Source: CAD feature listing. Evaluate the final solid. Frame: model axes, mm. A direction names the side the tool comes from. Round coordinates to 2 decimals unless told otherwise and drop trailing zeros. Loops run counter-clockwise (first coordinate to the right, second up) from the corner with the lowest first, then second, coordinate; pieces in that order, holes last. Notation, with made-up numbers: (50.5, -39) -> (57.5, -39) arc R28 cw to (57.5, -8) -> close; hole circle Ø8 at (16.5, 84). An arc over 180 degrees is marked (long way). Put each result on its own line as item: value. Start each with the question number.
1. Cut plane B-B (z = -37.5). Return the cut outline in (x, y).
2. Cut plane A-A (x = -4.25). Return the cut outline in (y, z), then the cut area to 3 significant figures.
3. Contact query for flat-ended pins moving along their axis: pin 1 (5 mm diameter, centred on x = -16.5, y = 26, fed in from -Z); pin 2 (9 mm diameter, centred on x = -9, z = -22, fed in from +Y); pin 3 (10 mm diameter, centred on x = -9, y = 17.5, fed in from +Z); pin 4 (4 mm diameter, centred on x = -13, z = -43, fed in from +Y). Output: stop coordinate, or through.
4. Cut plane C-C (z = -43). Return the cut outline in (x, y), then the cut area to 3 significant figures.
5. Set-up query: faces 1 (the flat face through (-10, 18, -40)), 2 (the cylindrical face through (-9.67, 43.21, -32.38)), 3 (the flat face through (-10, 18, 0)). Return all of +Z, -Z, +X, -X, +Y, -Y with unobstructed straight access to the full face (end or side cutting, diameter ignored); none if empty.
6. Material intervals for L1, parallel to X at y = 29.5, z = 4.75; L2, parallel to Y at x = -1, z = -36; L3, parallel to Y at x = -1.25, z = 1, sorted ascending.
7. Cut plane D-D (x = -10). Return the cut outline in (y, z), then the cut area to 3 significant figures.
Autodesk Inventor part; units mm, degrees
ref_plane "YZ Plane" through (0, 0, 0) normal (1, 0, 0) x (0, 1, 0)
ref_plane "XZ Plane" through (0, 0, 0) normal (0, 1, 0) x (-1, 0, 0)
ref_plane "XY Plane" through (0, 0, 0) normal (0, 0, 1) x (1, 0, 0)
sketch "Sketch1" plane through (0, 0, 0) normal (1, 0, 0) x (0, 1, 0)
  line L0 (0, 0) -> (40.5, 0)
  line L1 (40.5, 0) -> (40.5, -40)
  line L2 (40.5, -40) -> (0, -40)
  line L3 (0, -40) -> (0, 0)
  line L4 (46, -27.4) -> (40.5, -27.4)
  line L5 (40.5, -27.4) -> (40.5, -32.4)
  line L6 (40.5, -32.4) -> (46, -32.4)
  line L7 (46, -32.4) -> (46, -27.4)
  line L8 (46, -27.4) -> (40.5, -32.4) construction
  line L9 (40.5, -27.4) -> (46, -32.4) construction
  line L10 (40.5, -20) -> (0, -20) construction
  line L11 (27.5, 0) -> (30.5, 0)
  line L12 (30.5, 0) -> (30.5, 7.25)
  line L13 (30.5, 7.25) -> (27.5, 7.25)
  line L14 (27.5, 7.25) -> (27.5, 0)
  line L15 (27.5, -40) -> (30.5, -40)
  line L16 (30.5, -40) -> (30.5, -47.25)
  line L17 (30.5, -47.25) -> (27.5, -47.25)
  line L18 (27.5, -47.25) -> (27.5, -40)
  line L19 (3, -40) -> (6.5, -40)
  line L20 (6.5, -40) -> (6.5, -45.5)
  line L21 (6.5, -45.5) -> (3, -45.5)
  line L22 (3, -45.5) -> (3, -40)
  line L23 (0, -40) -> (7.5, -40)
  line L24 (7.5, -40) -> (7.5, 0)
  line L25 (7.5, 0) -> (0, 0)
  line L26 (0, 0) -> (0, -40)
  point P0 (43.25, -29.9)
  point P1 (30.5, 0)
  dimension "d0" = 40
  dimension "d1" = 40.5
  dimension "d2" = 10.1
  dimension "d3" = 5.5
  dimension "d4" = 5
  dimension "d5" = 20
  dimension "d6" = 3
  dimension "d7" = 27.5
  dimension "d8" = 7.25
  dimension "d31" = 3.5
  dimension "d32" = 5.5
  dimension "d33" = 21
  dimension "d34" = 3
  dimension "d41" = 3
  dimension "d42" = 20
  dimension "d43" = 7.5
sketch "Sketch2" plane through (0, 0, 0) normal (0, 1, 0) x (-1, 0, 0)
  line L0 (0, 0) -> (20, 0)
  line L1 (20, 0) -> (20, -40)
  line L2 (20, -40) -> (0, -40)
  line L3 (0, -40) -> (0, 0)
  line L4 (0, 0) -> (20, 0)
  line L5 (20, 0) -> (20, 7.25)
  line L6 (20, 7.25) -> (0, 7.25)
  line L7 (0, 7.25) -> (0, 0)
  circle A0 centre (5, 4.75) radius 2.5
  line L8 (10, 7.25) -> (10, 0) construction
  circle A1 centre (15, 4.75) radius 2.5
  line L9 (20, -20) -> (0, -20) construction
  line L10 (20, -40) -> (20, -47.25)
  line L11 (20, -47.25) -> (0, -47.25)
  line L12 (0, -47.25) -> (0, -40)
  circle A2 centre (5, -44.75) radius 2.5
  circle A3 centre (15, -44.75) radius 2.5
  circle A4 centre (10, -29.9) radius 2.5
  line L13 (0, -0.5) -> (19.5, -0.5)
  line L14 (19.5, -0.5) -> (19.5, -39.5)
  line L15 (19.5, -39.5) -> (0, -39.5)
  line L16 (0.5, -40) -> (0.5, 0)
  point P0 (0.5, -0.5)
  point P1 (0.5, -39.5)
  dimension "d9" = 40
  dimension "d10" = 20
  dimension "d11" = 7.25
  dimension "d12" = 20
  dimension "d13" = 5
  dimension "d14" = 5
  dimension "d15" = 2.5
  dimension "d16" = 5
  dimension "d17" = 10.1
  dimension "d18" = 10
  dimension "d19" = 14.85
  dimension "d20" = 34.65
  dimension "d21" = 54.5
  dimension "d30" = 49.5
  dimension "d44" = 0.5
  dimension "d45" = 0.5
extrude "Extrusion1" add sketch "Sketch1" against normal blind 20 contours L0 L1 L2 L24 | L14 L13 L12 L0 | L2 L16 L17 L18
extrude "Extrusion2" cut sketch "Sketch2" along normal blind 100 contours A1 | A0 | A2 | A3
extrude "Extrusion3" add sketch "Sketch2" along normal blind 46 contours A4
fillet "Fillet1" radius 2 4 edges at (-20, 29, 7.25) (0, 29, 7.25) (0, 29, -47.25) (-20, 29, -47.25)
fillet "Fillet2" radius 1 12 edges at (0, 17.5, 0) (0, 35.5, 0) (0, 35.5, -40) (0, 17.5, -40) (-20, 35.5, -40) (-20, 17.5, -40) (-20, 35.5, 0) (-20, 17.5, 0) (-20, 40.5, -20) (-10, 40.5, 0) (0, 40.5, -20) (-10, 40.5, -40)
extrude "Extrusion5" cut sketch "Sketch2" along normal blind 8.5 contours L0 L16 L13 L3 | L0 L1 L2 L16 L15 L14 L13 | L13 L16 L15 L3 | L15 L16 L2 L3
properties part number "Servo40KgRough"
Solution:
1. outline: (-20, 8.5) -> (-19.5, 8.5) -> (-19.5, 7.5) -> (-0.5, 7.5) -> (-0.5, 8.5) -> (0, 8.5) -> (0, 39.5) arc R1 ccw to (-1, 40.5) -> (-19, 40.5) arc R1 ccw to (-20, 39.5) -> close
2. outline: (7.5, -39.5) -> (8.5, -39.5) -> (8.5, -40) -> (27.5, -40) -> (27.5, -42.37) -> (30.5, -42.37) -> (30.5, -40) -> (39.5, -40) arc R1 ccw to (40.5, -39) -> (40.5, -1) arc R1 ccw to (39.5, 0) -> (30.5, 0) -> (30.5, 2.37) -> (27.5, 2.37) -> (27.5, 0) -> (8.5, 0) -> (8.5, -0.5) -> (7.5, -0.5) -> close; (27.5, -47.25) -> (30.5, -47.25) -> (30.5, -47.13) -> (27.5, -47.13) -> close; (27.5, 7.13) -> (30.5, 7.13) -> (30.5, 7.25) -> (27.5, 7.25) -> close
2. area: 1,330 mm^2
3. pin 1: stops at z = -47.25
3. pin 2: stops at y = 40.5
3. pin 3: stops at z = 0
3. pin 4: stops at y = 30.5
4. outline: (-20, 27.5) -> (-16.79, 27.5) -> (-16.79, 30.5) -> (-20, 30.5) -> close; (-13.21, 27.5) -> (-6.79, 27.5) -> (-6.79, 30.5) -> (-13.21, 30.5) -> close; (-3.21, 27.5) -> (0, 27.5) -> (0, 30.5) -> (-3.21, 30.5) -> close
4. area: 38.6 mm^2
5. face 1: -Z, +X, -X, -Y
5. face 2: +Y
5. face 3: +Z, +X, -X, -Y
6. L1: x = -20 to -17.5, -12.5 to -7.5, -2.5 to 0
6. L2: y = 7.5 to 40.5
6. L3: y = 27.5 to 30.5
7. outline: (0, -32.4) -> (7.5, -32.4) -> (7.5, -39.5) -> (8.5, -39.5) -> (8.5, -40) -> (27.5, -40) -> (27.5, -47.25) -> (30.5, -47.25) -> (30.5, -40) -> (39.5, -40) arc R1 ccw to (40.5, -39) -> (40.5, -32.4) -> (46, -32.4) -> (46, -27.4) -> (40.5, -27.4) -> (40.5, -1) arc R1 ccw to (39.5, 0) -> (30.5, 0) -> (30.5, 7.25) -> (27.5, 7.25) -> (27.5, 0) -> (8.5, 0) -> (8.5, -0.5) -> (7.5, -0.5) -> (7.5, -27.4) -> (0, -27.4) -> close
7. area: 1,430 mm^2
